CAD build for the part. Positions are in the model's coordinates, mm. A direction names the side the tool comes from. Coordinates: 2 decimals unless noted, no trailing zeros. Write each loop counter-clockwise with the first axis right and the second up, starting at its lowest first coordinate (ties: lowest second). Pieces come first, ordered by that corner, then holes. Notation, with made-up numbers: (15.5, -22.75) -> (31.5, -22.75) arc R26 ccw to (31.5, -6.75) -> close; hole circle Ø2 at (4, 84.25). An arc over 180 degrees is marked (long way). Answer as CSV lines item,"result". Start each with the question number.
```python
from build123d import *

# Parameters (mm, degrees)
F0_R     = 1.016
F0_R_2   = 1.905
F1_DEPTH = 3.175
F2_R     = 1.6002


with BuildPart() as f1:
    # F0 (on Top) → F1 (new body)
    with BuildSketch(Plane.XY):
        with BuildLine():
            Line((19.05, 7.9248), (19.05, 0))
            Line((19.05, 0), (65.0748, 0))
            ThreePointArc((65.0748, 0), (66.206312, 0.468688), (66.675, 1.6002))
            Line((66.675, 1.6002), (66.675, 30.1498))
            ThreePointArc((66.675, 30.1498), (66.206312, 31.281312), (65.0748, 31.75))
            Line((65.0748, 31.75), (1.6002, 31.75))
            ThreePointArc((1.6002, 31.75), (0.468688, 31.281312), (0, 30.1498))
            Line((0, 30.1498), (0, 9.525))
            Line((0, 9.525), (17.4498, 9.525))
            ThreePointArc((17.4498, 9.525), (18.581312, 9.056312), (19.05, 7.9248))
        make_face()
        with Locations((6.35, 15.875)):
            Circle(F0_R, mode=Mode.SUBTRACT)
        with Locations((40.386, 15.875)):
            Circle(F0_R_2, mode=Mode.SUBTRACT)
    extrude(amount=F1_DEPTH)

    # F2
    f2_edges = [f1.edges().sort_by_distance(p)[0] for p in [
        (0, 9.525, 1.5875),
        (19.05, 0, 1.5875),
    ]]
    fillet(f2_edges, radius=F2_R)


solid = f1.part
```
1. Cut at B-B (z = 0.75). Give the cut face in (x, y) (3 decimals).
2. Mould opens along X. For faces 1 (the face through (33, 16, 0)), 2 (the face through (6.218, 16.882, 1.565)), 3 (the face through (19.05, 5, 2)) say: pulls with the +X half, pulls with the -X half, needs draft (parallel to the pull), parting line crosses it, or undercut.
3. Cut at A-A (x = 6.35). Give the cut face in (y, z) (3 decimals).
4. Wall check: line 1 (Y direction, x = 6.35, z = 0.9) (3 decimals); line 2 (X direction, y = 7, z = 2.75) (3 decimals); line 3 (X direction, y = 10.5, z = 0.8) (3 decimals). Give the ranges that are in metal, low to high.
5. Cut at C-C (y = 3). Give the cut face in (x, z) (3 decimals).
6. Tool access for faces 4 (the face through (0, 21, 2)), 5 (the face through (9, 9.525, 2)): list every direction of +Z, -Z, +X, -X, +Y, -Y with a clear straight run to the whole face (end or side of a thin tool).
7. Flat gauge pins, fed straight in: P1, Ø1, axis at y = 5.5, z = 1.5, coming from the -X side; P2, Ø1, axis at x = 12.5, z = 2, coming from the -Y side (3 decimals). Where does each tip first touch, or does it go through?
Geometry check:
1,outline,"(0, 11.125) arc R1.6 ccw to (1.6, 9.525) -> (17.45, 9.525) arc R1.6 cw to (19.05, 7.925) -> (19.05, 1.6) arc R1.6 ccw to (20.65, 0) -> (65.075, 0) arc R1.6 ccw to (66.675, 1.6) -> (66.675, 30.15) arc R1.6 ccw to (65.075, 31.75) -> (1.6, 31.75) arc R1.6 ccw to (0, 30.15) -> close; hole circle Ø2.032 at (6.35, 15.875); hole circle Ø3.81 at (40.386, 15.875)"
2,face 1,"needs draft"
2,face 2,"undercut"
2,face 3,"pulls with the -X half"
3,outline,"(9.525, 0) -> (14.859, 0) -> (14.859, 3.175) -> (9.525, 3.175) -> close; (16.891, 0) -> (31.75, 0) -> (31.75, 3.175) -> (16.891, 3.175) -> close"
4,line 1,"9.525 to 14.859, 16.891 to 31.75"
4,line 2,"19.05 to 66.675"
4,line 3,"0.127 to 66.675"
5,outline,"(19.05, 0) -> (66.675, 0) -> (66.675, 3.175) -> (19.05, 3.175) -> close"
6,face 4,"+Z, -Z, -X, +Y, -Y"
6,face 5,"+Z, -Z, -X, -Y"
7,P1,"x = 19.05"
7,P2,"y = 9.525"
